```python
from build123d import *

# Parameters (mm, degrees)
SKETCH_3_W          = 33
SKETCH_3_H          = 22.7
EXTRUDE_2_DEPTH     = 6
SKETCH_4_W          = 14.3
SKETCH_4_H          = 4
EXTRUDE_3_DEPTH     = 12.7
SKETCH_5_R          = 2.5
CUT_EXTRUDE_2_DEPTH = 45.203845987
SKETCH_6_R          = 2.5
CUT_EXTRUDE_3_DEPTH = 40.924679084
SKETCH_7_W          = 12.7
SKETCH_7_H          = 3.5
EXTRUDE_4_DEPTH     = 6
EXTRUDE_START       = 3
SKETCH_8_W          = 12
SKETCH_8_H          = 24.7
SKETCH_8_R          = 2.5
EXTRUDE_5_DEPTH     = 3
EXTRUDE_6_DEPTH     = 3


with BuildPart() as part:
    # 草图3 → 凸台-拉伸2 (new body)
    with BuildSketch(Plane(origin=(0, 0, 0), x_dir=(1, 0, 0), z_dir=(0, 1, 0))):
        with Locations((16.5, 11.35)):
            Rectangle(SKETCH_3_W, SKETCH_3_H)
    extrude(amount=EXTRUDE_2_DEPTH)

    # 草图4 → 凸台-拉伸3 (add)
    with BuildSketch(Plane(origin=(0, 6, 0), x_dir=(1, 0, 0), z_dir=(0, 1, 0))):
        with Locations((25.85, 2)):
            Rectangle(SKETCH_4_W, SKETCH_4_H)
        Polygon((0, 0), (6, 0), (6, 16.7), (33, 16.7), (33, 22.7), (0, 22.7), align=None)
    extrude(amount=EXTRUDE_3_DEPTH)

    # 草图5 → 切除-拉伸2 (cut, through all)
    with BuildSketch(Plane.XY):
        with Locations((26.33, 12.35)):
            Circle(SKETCH_5_R)
    extrude(amount=-CUT_EXTRUDE_2_DEPTH, mode=Mode.SUBTRACT)

    # 草图6 → 切除-拉伸3 (cut, through all)
    with BuildSketch(Plane(origin=(6, 0, 0), x_dir=(0, 0, -1), z_dir=(1, 0, 0))):
        with Locations((9.07, 12.35)):
            Circle(SKETCH_6_R)
    extrude(amount=-CUT_EXTRUDE_3_DEPTH, mode=Mode.SUBTRACT)

    # 草图7 → 凸台-拉伸4 (add)
    with BuildSketch(Plane(origin=(0, 18.7, 0), x_dir=(1, 0, 0), z_dir=(0, 1, 0))):
        Polygon((0, 22.7), (0, 0), (6, 0), (6, 13.2), (6, 16.7), (18.7, 16.7), (18.7, 22.7), align=None)
        Polygon((33, 22.7), (18.7, 22.7), (18.7, 16.7), (22.2, 16.7), (33, 16.7), align=None)
        Polygon((22.2, 16.7), (18.7, 16.7), (18.7, 13.2), (18.7, 4), (18.7, 0), (33, 0), (33, 4), (22.2, 4), align=None)
        with Locations((12.35, 14.95)):
            Rectangle(SKETCH_7_W, SKETCH_7_H)
    extrude(amount=EXTRUDE_4_DEPTH)

    # 草图8 → 凸台-拉伸5 (add)
    with BuildSketch(Plane.XY.offset(EXTRUDE_START)):
        with Locations((27, 12.35)):
            Rectangle(SKETCH_8_W, SKETCH_8_H)
        with Locations((26.33, 12.35)):
            Circle(SKETCH_8_R, mode=Mode.SUBTRACT)
    extrude(amount=-EXTRUDE_5_DEPTH)

    # 草图9 → 凸台-拉伸6 (add)
    with BuildSketch(Plane.XY):
        Polygon((0, 24.7), (0, 0), (21, 0), (21, 4), (4, 4), (4, 24.7), align=None)
    extrude(amount=EXTRUDE_6_DEPTH)


solid = part.part
```
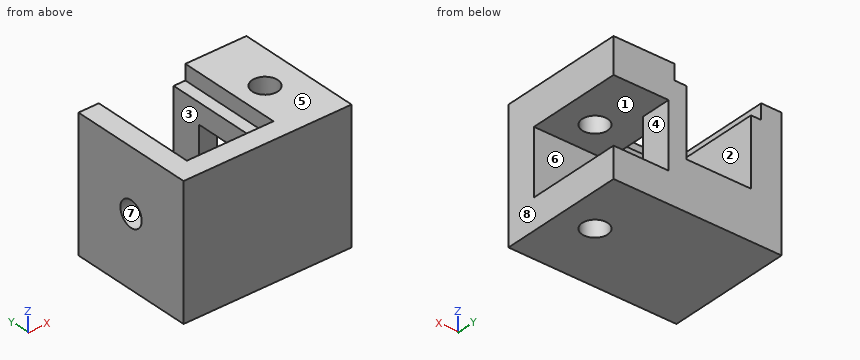
Geometry: final body of the model. Coordinates: model frame, mm. Face numbers are marked on the shaded views. A direction names the side the tool comes from. Round coordinates to 2 decimals unless told otherwise and drop trailing zeros. Order: outer loops, then holes, each group sorted by start corner. A loop starts at its lowest first (then second) coordinate and runs counter-clockwise, first axis right, second up. Notation, with made-up numbers: (-9.75, 62) -> (10.25, 62) arc R11 ccw to (10.25, 73) -> close; hole circle Ø9 at (83, -30.75). An arc over 180 degrees is marked (long way). Write each question's results on one line, items separated by ' | '.
Q1. Pin query (flat end, axial travel): pin 1 Ø3 at (x, y) = (8.5, 20.5) entering from +Z; pin 2 Ø3 at (y, z) = (20.5, -11) entering from +X; pin 3 Ø3.5 at (x, z) = (13.5, 1) entering from +Y. Return the tip coordinate at first contact, or that it passes through.
Response values:
pin 1: z = -13.2 | pin 2: x = 22.2 | pin 3: y = 6
Q2. Section query D-D (x = 26.33). Output: boundary loops of the cut face in (y, z), and give its area (3 significant figures).
Response values:
outline: (0, -22.7) -> (9.85, -22.7) -> (9.85, -16.7) -> (6, -16.7) -> (6, -4) -> (9.85, -4) -> (9.85, 3) -> (0, 3) -> close; (14.85, -22.7) -> (24.7, -22.7) -> (24.7, -16.7) -> (14.85, -16.7) -> close; (14.85, -4) -> (24.7, -4) -> (24.7, 3) -> (14.85, 3) -> close | area: 332 mm²
Q3. Ray query, line 1 along Z through (x, y) = (22, 7.5); line 2 along Y through (x, z) = (2.95, -9.07); line 3 along X through (y, z) = (8.25, -0.75). Return the intervals inside material, ascending.
Response values:
line 1: -22.7 to -16.7, -4 to 3 | line 2: 0 to 9.85, 14.85 to 24.7 | line 3: 0 to 6, 18.7 to 33
Q4. Access query for the marked faces 1, 2, 3 and 4. Directions: +Z, -Z, +X, -X, +Y, -Y. A direction counts if a zero-diameter tool reaches every point of the face in a straight line with its end or side. Return the directions, or none.
Response values:
face 1: +X | face 2: +Z | face 3: +Z, +Y | face 4: +X, +Y
Q5. Section query C-C (y = 17.5). Output: boundary loops of the cut face in (x, z).
Response values:
outline: (0, -22.7) -> (33, -22.7) -> (33, -16.7) -> (6, -16.7) -> (6, 0) -> (4, 0) -> (4, 3) -> (0, 3) -> close; (18.7, -4) -> (33, -4) -> (33, 3) -> (21, 3) -> (21, 0) -> (18.7, 0) -> close
Q6. Section query B-B (y = 12.35). Output: boundary loops of the cut face in (x, z).
Response values:
outline: (0, -22.7) -> (23.83, -22.7) -> (23.83, -16.7) -> (6, -16.7) -> (6, -11.57) -> (0, -11.57) -> close; (0, -6.57) -> (6, -6.57) -> (6, 0) -> (4, 0) -> (4, 3) -> (0, 3) -> close; (18.7, -4) -> (23.83, -4) -> (23.83, 3) -> (21, 3) -> (21, 0) -> (18.7, 0) -> close; (28.83, -22.7) -> (33, -22.7) -> (33, -16.7) -> (28.83, -16.7) -> close; (28.83, -4) -> (33, -4) -> (33, 3) -> (28.83, 3) -> close
Q7. Section query A-A (z = -9.07). Output: boundary loops of the cut face in (x, y).
Response values:
outline: (0, 0) -> (33, 0) -> (33, 6) -> (6, 6) -> (6, 9.85) -> (0, 9.85) -> close; (0, 14.85) -> (6, 14.85) -> (6, 24.7) -> (0, 24.7) -> close; (18.7, 18.7) -> (22.2, 18.7) -> (22.2, 24.7) -> (18.7, 24.7) -> close
Q8. Pull-direction query (Z, two-part tool) for the marked faces 5, 6, 7 and 8; classes: released by +Z, released by -Z, zero draft, split by the parting line, or undercut.
Response values:
face 5: released by +Z | face 6: undercut | face 7: undercut | face 8: zero draft
